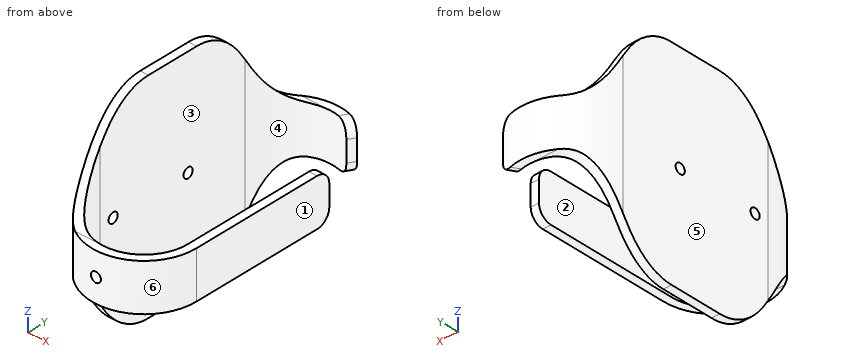
from build123d import *

# Parameters (mm, degrees)
HAND_BAND_BODY_DEPTH      = 41
HAND_BAND_BODY_DEPTH_BACK = 41
BACK_HAND_BRACE_DEPTH     = 93.092344959
PALM_BAND_OUTLINE_W       = 32
PALM_BAND_OUTLINE_H       = 100
PALM_BAND_DEPTH           = 20
SKETCH3_R                 = 1.89865
F_6_BOTTOM_HOLE_DEPTH     = 10
SKETCH4_R                 = 1.89865
F_6_SIDE_HOLES_DEPTH      = 20
FILLET1_R                 = 5


# Read off the part's stored shape, not the designer's step: Palm Band
with BuildPart() as part:
    # Sketch1 → Hand Band Body (new, two sides: drawn at the far end of the back side and taken through both)
    with BuildSketch(Plane.XY.offset(-HAND_BAND_BODY_DEPTH_BACK)):
        with BuildLine():
            Line((-20, 0), (-20, 60))
            ThreePointArc((-20, 60), (-10, 77.320508076), (10, 77.320508076))
            Line((10, 77.320508076), (8.4125, 74.570877419))
            ThreePointArc((8.4125, 74.570877419), (-8.4125, 74.570877419), (-16.825, 60))
            Line((-16.825, 60), (-16.825, 0))
            ThreePointArc((-16.825, 0), (0, -16.825), (16.825, 0))
            Line((16.825, 0), (16.825, 55))
            Line((16.825, 55), (20, 55))
            Line((20, 55), (20, 0))
            ThreePointArc((20, 0), (0, -20), (-20, 0))
        make_face()
    extrude(amount=HAND_BAND_BODY_DEPTH + HAND_BAND_BODY_DEPTH_BACK)

    # Sketch2 → Back-Hand Brace (cut, through all)
    with BuildSketch(Plane(origin=(0, 0, 0), x_dir=(0, 0, -1), z_dir=(1, 0, 0))):
        with BuildLine():
            Line((41, 80), (9, 80))
            Line((9, 80), (9, 76.825))
            add(Edge.make_bspline(
                [(9, 76.825), (9, 76.683054398), (9, 73.844142348), (17.85340715, 63.039379279), (34.522211451, 58.42224391), (41, 44.67531916), (41, 40.222634246), (41, 40)],
                knots=[0, 0, 0, 0, 0.008269556, 0.165391112, 0.746027462, 0.987301373, 1, 1, 1, 1], degree=3))
            Line((41, 40), (41, 80))
        make_face()
        with BuildLine():
            Line((41, -20), (41, 20))
            add(Edge.make_bspline(
                [(9, -16.825), (9, -16.683054398), (9, -13.844142348), (17.85340715, -3.039379279), (34.522211451, 1.57775609), (41, 15.32468084), (41, 19.777365754), (41, 20)],
                knots=[0, 0, 0, 0, 0.008269556, 0.165391112, 0.746027462, 0.987301373, 1, 1, 1, 1], degree=3))
            Line((9, -16.825), (9, -20))
            Line((9, -20), (41, -20))
        make_face()
        with BuildLine():
            Line((-41, 80), (-41, 40))
            add(Edge.make_bspline(
                [(-41, 40), (-41, 40.223460634), (-41, 44.692673321), (-34.522211451, 58.40583885), (-17.85340715, 63.020392952), (-9, 73.856007673), (-9, 76.683619413), (-9, 76.825)],
                knots=[0, 0, 0, 0, 0.012698627, 0.253972538, 0.834608888, 0.991730444, 1, 1, 1, 1], degree=3))
            Line((-9, 76.825), (-9, 80))
            Line((-9, 80), (-41, 80))
        make_face()
        with BuildLine():
            add(Edge.make_bspline(
                [(-9, -16.825), (-9, -16.683054398), (-9, -13.844142348), (-17.85340715, -3.039379279), (-34.522211451, 1.57775609), (-41, 15.32468084), (-41, 19.777365754), (-41, 20)],
                knots=[0, 0, 0, 0, 0.008269556, 0.165391112, 0.746027462, 0.987301373, 1, 1, 1, 1], degree=3))
            Line((-41, 20), (-41, -20))
            Line((-41, -20), (-9, -20))
            Line((-9, -20), (-9, -16.825))
        make_face()
    extrude(amount=-BACK_HAND_BRACE_DEPTH, mode=Mode.SUBTRACT)

    # Palm Band outline → Palm Band (cut)
    with BuildSketch(Plane(origin=(0, 0, 0), x_dir=(0, 0, -1), z_dir=(1, 0, 0))):
        with Locations((-25, 30)):
            Rectangle(PALM_BAND_OUTLINE_W, PALM_BAND_OUTLINE_H)
        with Locations((25, 30)):
            Rectangle(PALM_BAND_OUTLINE_W, PALM_BAND_OUTLINE_H)
    extrude(amount=PALM_BAND_DEPTH, mode=Mode.SUBTRACT)

    # Sketch3 → #6 Bottom Hole (cut)
    with BuildSketch(Plane(origin=(0, -25, 0), x_dir=(-1, 0, 0), z_dir=(0, 1, 0))):
        with Locations(Location((0, 0, 0), (0, 0, 270))):
            Circle(SKETCH3_R)
    extrude(amount=F_6_BOTTOM_HOLE_DEPTH, mode=Mode.SUBTRACT)

    # Sketch4 → #6 Side Holes (cut)
    with BuildSketch(Plane(origin=(-25, 0, 0), x_dir=(0, 0, -1), z_dir=(1, 0, 0))):
        with Locations(Location((0, 36.4, 0), (0, 0, 180))):
            Circle(SKETCH4_R)
        with Locations(Location((0, 5.4, 0), (0, 0, 180))):
            Circle(SKETCH4_R)
    extrude(amount=F_6_SIDE_HOLES_DEPTH, mode=Mode.SUBTRACT)

    # Fillet1
    fillet1_edges = [part.edges().sort_by_distance(p)[0] for p in [
        (18.4125, 55, -9),
        (9.20625, 75.945692747, -9),
        (9.20625, 75.945692747, 9),
        (18.4125, 55, 9),
    ]]
    fillet(fillet1_edges, radius=FILLET1_R)


solid = part.part
The model under review builds one solid part; all positions refer to its coordinate system, in mm. Face numbers are marked on the shaded views. A direction names the side the tool comes from. Round coordinates to 2 decimals unless told otherwise and drop trailing zeros. Loops run counter-clockwise (first coordinate to the right, second up) from the corner with the lowest first, then second, coordinate; pieces in that order, holes last. Notation, with made-up numbers: M 23.5,46.25 L 44.5,46.25 A31 cw 44.5,85.25 Z; hole C 58.5,-29.5 d2. An arc over 180 degrees is marked long. Answer as CSV lines item,"result".
1. Draft analysis for pull direction Y (two halves, no side actions). For the marked faces 4, 5 and 6, state which applies: pulls with the +Y half, pulls with the -Y half, needs draft (parallel to the pull), parting line crosses it, or undercut.
Outcome:
face 4,"undercut"
face 5,"needs draft"
face 6,"pulls with the -Y half"
2. We need section B-B (z = 0). Count the separate pieces of the cut face and the enclosed holes in it, plus the area to 3 significant figures.
Outcome:
separate pieces,"4"
enclosed holes,"0"
area,"635 mm2"
3. We need section A-A (y = 36.4). Give the boundary of the cut face in (x, z) (3 decimals).
Outcome:
outline,"M -20,-41 L -16.825,-41 L -16.825,-1.899 L -20,-1.899 Z; M -20,1.899 L -16.825,1.899 L -16.825,41 L -20,41 Z; M 16.825,-9 L 20,-9 L 20,9 L 16.825,9 Z"
4. For the marked faces 1, 2 and 3, list the 3-axis set-ups (+Z, -Z, +X, -X, +Y, -Y) from which the entire face can be reached by the end or side of a thin tool; tool diameter is ignored.
Outcome:
face 1,"+Z, -Z, +X, +Y, -Y"
face 2,"+Z, -Z, +Y"
face 3,"+Z, -Z"
5. Insertion check: pin 1 Ø4 at (x, y) = (1, 78.5) entering from -Z; pin 2 Ø1.5 at (x, z) = (-9.5, 4) entering from -Y; pin 3 Ø8 at (x, z) = (4.5, -6) entering from -Y. Each pin has a flat end and moves straight along its axis. Give the tip position at first contact, or say it passes through.
Outcome:
pin 1,"stops at z = -9"
pin 2,"stops at y = -17.98"
pin 3,"stops at y = -19.99"
6. To check wall thickness, follow L1, parallel to Y at x = -18, z = 0; L2, parallel to X at y = 44, z = 4.5 (3 decimals); L3, parallel to X at y = 43, z = -10.5 (3 decimals). State the ranges of each line that lie inside material, in increasing order. Write a range as [from, to].
Outcome:
L1,"y = [-8.72, 3.5], [7.3, 34.5], [38.3, 68.72]"
L2,"x = [-20, -16.825], [16.825, 20]"
L3,"x = [-20, -16.825]"
7. We need section C-C (x = 13). Give the boundary of the cut face in (y, z), plus the area to 3 significant figures.
Outcome:
outline,"M -15.2,-9 L -10.68,-9 L -10.68,9 L -15.2,9 Z"
area,"81.3 mm2"
